from build123d import *

# Parameters (mm, degrees)
EXTRUDE_1_DEPTH = 3


with BuildPart() as part:
    # 草圖1 → 填料-伸長1 (new body)
    with BuildSketch(Plane.XY):
        with BuildLine():
            Line((-5, 40), (-15, 40))
            ThreePointArc((-15, 40), (-32.67766953, 32.67766953), (-40, 15))
            Line((-40, 15), (-40, 5))
            Line((-40, 5), (-37, 5))
            Line((-37, 5), (-37, -5))
            Line((-37, -5), (-40, -5))
            Line((-40, -5), (-40, -15))
            ThreePointArc((-40, -15), (-32.67766953, -32.67766953), (-15, -40))
            Line((-15, -40), (-5, -40))
            Line((-5, -40), (-5, -37))
            Line((-5, -37), (5, -37))
            Line((5, -37), (5, -40))
            Line((5, -40), (15, -40))
            ThreePointArc((15, -40), (32.67766953, -32.67766953), (40, -15))
            Line((40, -15), (40, -5))
            Line((40, -5), (37, -5))
            Line((37, -5), (37, 5))
            Line((37, 5), (40, 5))
            Line((40, 5), (40, 15))
            ThreePointArc((40, 15), (32.67766953, 32.67766953), (15, 40))
            Line((15, 40), (5, 40))
            Line((5, 40), (5, 37))
            Line((5, 37), (-5, 37))
            Line((-5, 37), (-5, 40))
        make_face()
    extrude(amount=EXTRUDE_1_DEPTH)


solid = part.part
Design review of the part built by this model. Coordinates are the model's own, in mm. A direction names the side the tool comes from. Round coordinates to 2 decimals unless told otherwise and drop trailing zeros. Write each loop counter-clockwise with the first axis right and the second up, starting at its lowest first coordinate (ties: lowest second). Pieces come first, ordered by that corner, then holes. Notation, with made-up numbers: (-3, 15.5) - (26, 15.5) arc R15 ccw to (26, 37.5) - close; hole circle Ø11 at (78, 68). An arc over 180 degrees is marked (long way). Use a Markdown table: item, result. Add a question column.
1. Mouldability with a two-part tool opening along Y and no side actions: class faces 5 (the face through (40, 10, 1)), 6 (the face through (38, 5, 1)), 7 (the face through (-32.482, 32.871, 1.479)) as +Y half, -Y half, draft (parallel to the pull), parting line (faces both ways), or undercut.
2. Clearance check with flat-ended pins moving along their axes: pin 1 (0.9 mm diameter, centred on y = -1, z = 1.5, fed in from +X); pin 2 (1.5 mm diameter, centred on y = 0.5, z = 1.5, fed in from -X); pin 3 (0.9 mm diameter, centred on x = 2, z = 1, fed in from -Y). State where each tip first meets the part, or that it passes through.
3. Wall thickness on probe 1 along Y at (x, z) = (1.5, 2.85); probe 2 along Y at (x, z) = (-16.5, 1.25): over which ranges is each line inside the solid? List them lowest first.
4. We need section C-C (y = 26.5). State the section outline as (x, z) points.
5. We need section B-B (x = 22). State the section outline as (y, z) points, then the cut area to 3 significant figures.
6. We need section A-A (z = 1.45). State the section outline as (x, y) points.
7. For faces 1 (the face through (0, -37, 1)), 2 (the face through (-37, 0, 1)), 3 (the face through (-40, 10, 1)), 4 (the face through (5, 39, 1)), list the 3-axis set-ups (+Z, -Z, +X, -X, +Y, -Y) from which the entire face can be reached by the end or side of a thin tool; tool diameter is ignored.
Output:
| question | item | result |
|---|---|---|
| 1 | face 5 | draft |
| 1 | face 6 | undercut |
| 1 | face 7 | +Y half |
| 2 | pin 1 | stops at x = 37 |
| 2 | pin 2 | stops at x = -37 |
| 2 | pin 3 | stops at y = -37 |
| 3 | probe 1 | y = -37 to 37 |
| 3 | probe 2 | y = -39.95 to 39.95 |
| 4 | outline | (-37.2, 0) - (37.2, 0) - (37.2, 3) - (-37.2, 3) - close |
| 5 | outline | (-39, 0) - (39, 0) - (39, 3) - (-39, 3) - close |
| 5 | area | 234 mm2 |
| 6 | outline | (-40, -15) arc R25 ccw to (-15, -40) - (-5, -40) - (-5, -37) - (5, -37) - (5, -40) - (15, -40) arc R25 ccw to (40, -15) - (40, -5) - (37, -5) - (37, 5) - (40, 5) - (40, 15) arc R25 ccw to (15, 40) - (5, 40) - (5, 37) - (-5, 37) - (-5, 40) - (-15, 40) arc R25 ccw to (-40, 15) - (-40, 5) - (-37, 5) - (-37, -5) - (-40, -5) - close |
| 7 | face 1 | +Z, -Z, -Y |
| 7 | face 2 | +Z, -Z, -X |
| 7 | face 3 | +Z, -Z, -X, +Y, -Y |
| 7 | face 4 | +Z, -Z, +Y |
